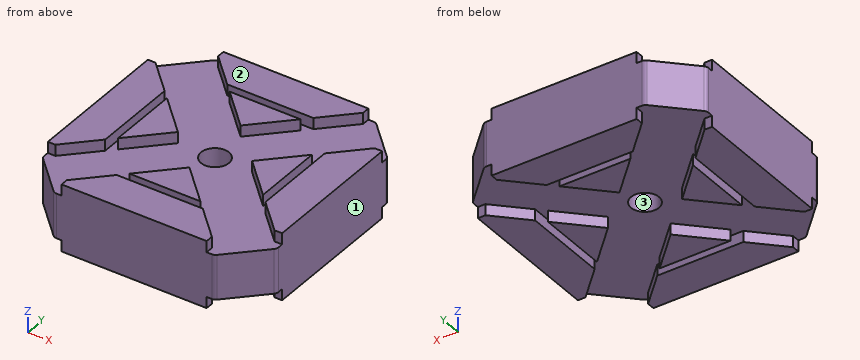
from build123d import *

# Parameters (mm, degrees)
BOSS_EXTRUDE1_DEPTH = 6
SKETCH2_W           = 1.355339059
SKETCH2_H           = 2
CUT_EXTRUDE1_DEPTH  = 43
SKETCH3_W           = 2
SKETCH3_H           = 1.355339059
CUT_EXTRUDE2_DEPTH  = 43
SKETCH4_W           = 2
SKETCH4_H           = 9.39696962
CUT_EXTRUDE3_DEPTH  = 55.69848481
SKETCH5_W           = 2
SKETCH5_H           = 9.39696962
CUT_EXTRUDE4_DEPTH  = 55.69848481
SKETCH7_R           = 2.5
CUT_EXTRUDE7_DEPTH  = 7
FILLET1_R           = 1


with BuildPart() as part:
    # Sketch1 → Boss-Extrude1 (new body)
    with BuildSketch(Plane.XY):
        Polygon((-21, 14.355339059), (-14.355339059, 21), (14.355339059, 21), (21, 14.355339059), (21, -14.355339059), (14.355339059, -21), (-14.355339059, -21), (-21, -14.355339059), align=None)
    boss_extrude1 = extrude(amount=BOSS_EXTRUDE1_DEPTH)

    # Sketch2 → Cut-Extrude1 (cut, through all)
    with BuildSketch(Plane(origin=(0, 21, 0), x_dir=(1, 0, 0), z_dir=(0, 1, 0))):
        with Locations((-13.67766953, -1)):
            Rectangle(SKETCH2_W, SKETCH2_H)
        with Locations((13.67766953, -1)):
            Rectangle(SKETCH2_W, SKETCH2_H)
    cut_extrude1 = extrude(amount=-CUT_EXTRUDE1_DEPTH, mode=Mode.SUBTRACT)

    # Sketch3 → Cut-Extrude2 (cut, through all)
    with BuildSketch(Plane.ZY.offset(21)):
        with Locations((1, 13.67766953)):
            Rectangle(SKETCH3_W, SKETCH3_H)
        with Locations((1, -13.67766953)):
            Rectangle(SKETCH3_W, SKETCH3_H)
    cut_extrude2 = extrude(amount=-CUT_EXTRUDE2_DEPTH, mode=Mode.SUBTRACT)

    # Sketch4 → Cut-Extrude3 (cut, through all)
    with BuildSketch(Plane(origin=(17.67766953, 17.67766953, 0), x_dir=(0, 0, -1), z_dir=(0.707106781, 0.707106781, 0))):
        with Locations((-1, 0)):
            Rectangle(SKETCH4_W, SKETCH4_H)
    cut_extrude3 = extrude(amount=-CUT_EXTRUDE3_DEPTH, mode=Mode.SUBTRACT)

    # Sketch5 → Cut-Extrude4 (cut, through all)
    with BuildSketch(Plane(origin=(-17.67766953, 17.67766953, 0), x_dir=(0, 0, 1), z_dir=(-0.707106781, 0.707106781, 0))):
        with Locations((1, 0)):
            Rectangle(SKETCH5_W, SKETCH5_H)
    cut_extrude4 = extrude(amount=-CUT_EXTRUDE4_DEPTH, mode=Mode.SUBTRACT)

    # Sketch7 → Cut-Extrude7 (cut, through all)
    with BuildSketch(Plane(origin=(0, 0, 0), x_dir=(-1, 0, 0), z_dir=(0, 0, -1))):
        Circle(SKETCH7_R)
    cut_extrude7 = extrude(amount=-CUT_EXTRUDE7_DEPTH, mode=Mode.SUBTRACT)

    # Mirror2: Boss-Extrude1, Cut-Extrude1, Cut-Extrude2, Cut-Extrude3, Cut-Extrude4, Cut-Extrude7 across plane
    add(boss_extrude1.mirror(Plane(origin=(0, 0, 6), x_dir=(1, 0, 0), z_dir=(0, 0, -1))))
    add(cut_extrude1.mirror(Plane(origin=(0, 0, 6), x_dir=(1, 0, 0), z_dir=(0, 0, -1))), mode=Mode.SUBTRACT)
    add(cut_extrude2.mirror(Plane(origin=(0, 0, 6), x_dir=(1, 0, 0), z_dir=(0, 0, -1))), mode=Mode.SUBTRACT)
    add(cut_extrude3.mirror(Plane(origin=(0, 0, 6), x_dir=(1, 0, 0), z_dir=(0, 0, -1))), mode=Mode.SUBTRACT)
    add(cut_extrude4.mirror(Plane(origin=(0, 0, 6), x_dir=(1, 0, 0), z_dir=(0, 0, -1))), mode=Mode.SUBTRACT)
    add(cut_extrude7.mirror(Plane(origin=(0, 0, 6), x_dir=(1, 0, 0), z_dir=(0, 0, -1))), mode=Mode.SUBTRACT)

    # Fillet1
    fillet1_edges = [part.edges().sort_by_distance(p)[0] for p in [
        (-14.355339059, 21, 6),
        (-14.355339059, -21, 6),
        (14.355339059, 21, 6),
        (14.355339059, -21, 6),
        (-21, 14.355339059, 6),
        (21, 14.355339059, 6),
        (21, -14.355339059, 6),
        (-21, -14.355339059, 6),
    ]]
    fillet(fillet1_edges, radius=FILLET1_R)


solid = part.part
Work out the finished part from the listing and answer in its coordinate system (mm). Face numbers are marked on the shaded views. Coordinates: 2 decimals unless noted, no trailing zeros. Write each loop counter-clockwise with the first axis right and the second up, starting at its lowest first coordinate (ties: lowest second). Pieces come first, ordered by that corner, then holes.
1. The part is cut by section D-D, the plane z = 10.5. State how many separate pieces and enclosed holes the cut face has, and give its area (3 significant figures).
Results list:
separate pieces: 8
enclosed holes: 0
area: 741 mm2
2. Flat-ended cylindrical pins translate along their axes: pin 1 (1.5 mm diameter, centred on x = 20, z = 1, fed in from +Y); pin 2 (1.5 mm diameter, centred on y = -20.5, z = 1.5, fed in from -X); pin 3 (1.5 mm diameter, centred on x = 15.5, y = -9.5, fed in from +Z); pin 4 (6 mm diameter, centred on x = 12, y = 10.5, fed in from -Z). Find the tip coordinate at first contact, or state that the pin passes through.
Results list:
pin 1: stops at y = 13
pin 2: stops at x = -15.41
pin 3: stops at z = 12
pin 4: stops at z = 2
3. Consider line 1 along X through (y, z) = (0, 6.25); line 2 along Y through (x, z) = (-0.5, 1.75). Determine where each line is inside the solid, lowest interval first.
Results list:
line 1: x = -21 to -2.5, 2.5 to 21
line 2: y = -21 to -14.36, -13 to -7.14, 7.14 to 13, 14.36 to 21
4. The part is cut by section A-A, the plane z = 7. Write down the section's boundary in (x, y).
Results list:
outline: (-21, -13.94) arc R1 ccw to (-20.71, -14.65) - (-14.65, -20.71) arc R1 ccw to (-13.94, -21) - (13.94, -21) arc R1 ccw to (14.65, -20.71) - (20.71, -14.65) arc R1 ccw to (21, -13.94) - (21, 13.94) arc R1 ccw to (20.71, 14.65) - (14.65, 20.71) arc R1 ccw to (13.94, 21) - (-13.94, 21) arc R1 ccw to (-14.65, 20.71) - (-20.71, 14.65) arc R1 ccw to (-21, 13.94) - close; hole circle Ø5 at (0, 0)
5. For a pull along X with two mould halves and no side action, classify the marked faces 1, 2 and 3 as +X half, -X half, draft (parallel to the pull), parting line (faces both ways), or undercut.
Results list:
face 1: +X half
face 2: draft
face 3: undercut
